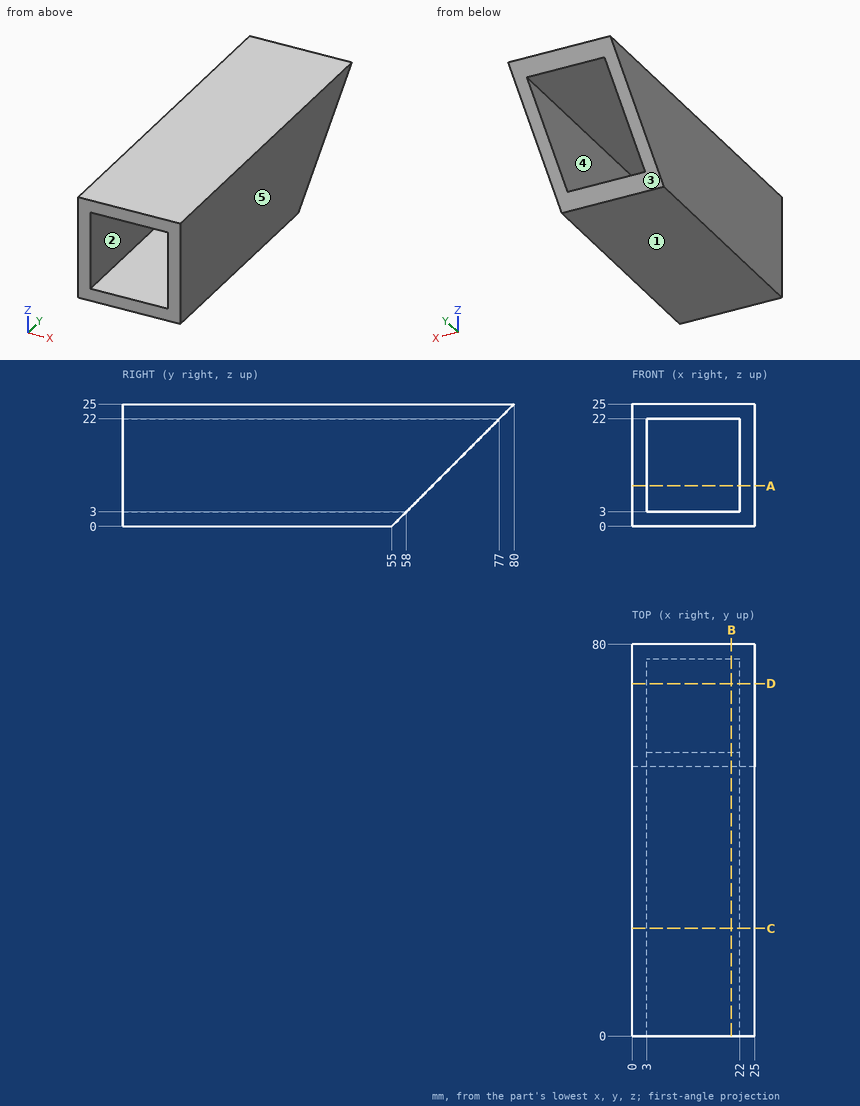
The figure shows three views and two pictorial views of one solid part (mm, origin at its lowest corner). Answer the questions. A direction names the side the tool comes from. Give positions to 0.01 mm unless a question says otherwise; leave off trailing zeros. Write each loop counter-clockwise with the first axis right and the second up, starting at its lowest first coordinate (ties: lowest second). Pieces come first, ordered by that corner, then holes. Notation, with made-up numbers: (-25.75, 89) - (-8.75, 89) arc R15 ccw to (-8.75, 95) - close; hole circle Ø4 at (79, -9). An arc over 180 degrees is marked (long way). Return JSON: item names as keys, results as strings.
Q1. For the marked faces 1 and 2, determine the directions among +Z, -Z, +X, -X, +Y, -Y from which every point of the face is accessible in a straight line to the end or side of a thin tool.
Reply:
{"face 1": "-Z, +X, -X, +Y, -Y", "face 2": "+Y, -Y"}
Q2. A cutting plane is placed at D-D, the plane y = 72. Determine the outline of the cut face in (x, z), and give its area (3 significant figures).
Reply:
{"outline": "(0, 17) - (3, 17) - (3, 22) - (22, 22) - (22, 17) - (25, 17) - (25, 25) - (0, 25) - close", "area": "105 mm²"}
Q3. A cutting plane is placed at A-A, the plane z = 8.25. Determine the outline of the cut face in (x, y).
Reply:
{"outline": "(0, 0) - (3, 0) - (3, 63.25) - (0, 63.25) - close; (22, 0) - (25, 0) - (25, 63.25) - (22, 63.25) - close"}
Q4. For a pull along X with two mould halves and no side action, classify the marked faces 3, 4 and 5 as released by +X, released by -X, zero draft, split by the parting line, or undercut.
Reply:
{"face 3": "zero draft", "face 4": "undercut", "face 5": "released by +X"}
Q5. A cutting plane is placed at B-B, the plane x = 20.25. Determine the outline of the cut face in (y, z).
Reply:
{"outline": "(0, 0) - (55, 0) - (58, 3) - (0, 3) - close; (0, 22) - (77, 22) - (80, 25) - (0, 25) - close"}
Q6. Consider line 1 along X through (y, z) = (52, 13.75); line 2 along Z through (x, y) = (19, 72). Determine where each line is inside the solid, lowest interval first. Write a range as [from, to].
Reply:
{"line 1": "[0, 3], [22, 25]", "line 2": "[22, 25]"}
Q7. A cutting plane is placed at C-C, the plane y = 22. Determine the outline of the cut face in (x, z).
Reply:
{"outline": "(0, 0) - (25, 0) - (25, 25) - (0, 25) - close; hole (3, 3) - (22, 3) - (22, 22) - (3, 22) - close"}
Q8. Given P1, Ø1, axis at x = 19.5, y = 64.5, coming from the -Z side, flat-ended and moving along its own axis, determine where the tip first touches the part or whether it passes through.
Reply:
{"P1": "z = 22"}
